Here's how the part is built. I have some questions about the finished solid (model axes, mm). Face numbers are marked on the shaded views. A direction names the side the tool comes from. Round coordinates to 2 decimals unless told otherwise and drop trailing zeros. Order: outer loops, then holes, each group sorted by start corner. A loop starts at its lowest first (then second) coordinate and runs counter-clockwise, first axis right, second up. Notation, with made-up numbers: (60, 11) - (79, 11) arc R21 ccw to (79, 16) - close; hole circle Ø9 at (49.25, 13). An arc over 180 degrees is marked (long way). Answer as a JSON object with one key per item and string values.
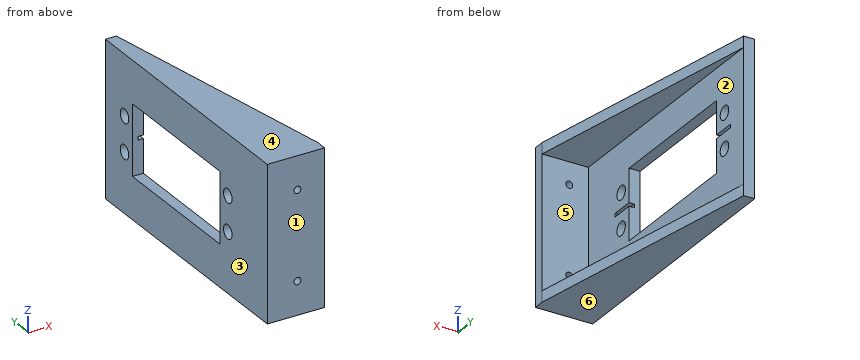
```python
from build123d import *

# Parameters (mm, degrees)
BOSS_EXTRUDE1_DEPTH = 22.225
BOSS_EXTRUDE2_DEPTH = 3.175
SKETCH4_R           = 1.000000032
CUT_EXTRUDE2_DEPTH  = 4.175
SKETCH5_R           = 2.000000064
CUT_EXTRUDE3_DEPTH  = 4.175
SKETCH6_W           = 20.253999878
SKETCH6_H           = 41.153999988
CUT_EXTRUDE4_DEPTH  = 4.175
SKETCH7_W           = 1.500000048
SKETCH7_H           = 1.000000032
CUT_EXTRUDE5_DEPTH  = 6.604
CUT_EXTRUDE6_START  = 41.154
SKETCH7_2_W         = 1.500000048
SKETCH7_2_H         = 1.000000032
CUT_EXTRUDE6_DEPTH  = 6.604


with BuildPart() as part:
    # Sketch1 → Boss-Extrude1 (new body, symmetric)
    with BuildSketch(Plane.XY):
        Polygon((0, 0), (0, 76.2), (3.175, 76.2), (3.175, 3.175), (16.51, 3.175), (16.51, 0), align=None)
    extrude(amount=BOSS_EXTRUDE1_DEPTH, both=True)

    # Sketch3 → Boss-Extrude2 (add)
    with BuildSketch(Plane.XY.offset(22.225)):
        Polygon((3.175, 76.2), (16.51, 3.175), (3.175, 3.175), align=None)
    boss_extrude2 = extrude(amount=-BOSS_EXTRUDE2_DEPTH)

    # Mirror1: Boss-Extrude2 across plane
    add(boss_extrude2.mirror(Plane.XY))

    # Sketch4 → Cut-Extrude2 (cut, through all)
    with BuildSketch(Plane(origin=(0, 3.175, 0), x_dir=(1, 0, 0), z_dir=(0, 1, 0))):
        with Locations((8.679999912, 12.7)):
            Circle(SKETCH4_R)
        with Locations((8.679999912, -12.7)):
            Circle(SKETCH4_R)
    extrude(amount=-CUT_EXTRUDE2_DEPTH, mode=Mode.SUBTRACT)

    # Sketch5 → Cut-Extrude3 (cut, through all)
    with BuildSketch(Plane(origin=(3.175, 0, 0), x_dir=(0, 0, -1), z_dir=(1, 0, 0))):
        with Locations((-4.953, 18.574999934)):
            Circle(SKETCH5_R)
        with Locations((5.047000066, 18.574999934)):
            Circle(SKETCH5_R)
        with Locations((-4.953, 67.175000016)):
            Circle(SKETCH5_R)
        with Locations((5.047000066, 67.175000016)):
            Circle(SKETCH5_R)
    extrude(amount=-CUT_EXTRUDE3_DEPTH, mode=Mode.SUBTRACT)

    # Sketch6 → Cut-Extrude4 (cut, through all)
    with BuildSketch(Plane(origin=(3.175, 0, 0), x_dir=(0, 0, -1), z_dir=(1, 0, 0))):
        with Locations((0.047000033, 42.874999975)):
            Rectangle(SKETCH6_W, SKETCH6_H)
    extrude(amount=-CUT_EXTRUDE4_DEPTH, mode=Mode.SUBTRACT)

    # Sketch7 → Cut-Extrude5 (cut)
    with BuildSketch(Plane.XZ.offset(-63.451999969)):
        with Locations((2.424999976, 0)):
            Rectangle(SKETCH7_W, SKETCH7_H)
    extrude(amount=-CUT_EXTRUDE5_DEPTH, mode=Mode.SUBTRACT)

    # Sketch7<2> → Cut-Extrude6 (cut)
    with BuildSketch(Plane.XZ.offset(-63.451999969).offset(CUT_EXTRUDE6_START)):
        with Locations((2.424999976, 0)):
            Rectangle(SKETCH7_2_W, SKETCH7_2_H)
    extrude(amount=CUT_EXTRUDE6_DEPTH, mode=Mode.SUBTRACT)


solid = part.part
```
1. Imagine slicing it at C-C (z = 12.7). List the corners of the cut face in (x, y) for me (3 decimals).
Responses:
{"outline": "(0, 0) - (7.68, 0) - (7.68, 3.175) - (3.175, 3.175) - (3.175, 76.2) - (0, 76.2) - close; (9.68, 0) - (16.51, 0) - (16.51, 3.175) - (9.68, 3.175) - close"}
2. For P1, Ø1.1, axis at y = 66, z = 0, coming from the +X side (3 decimals); P2, Ø3, axis at x = 8.68, z = 12.7, coming from the +Y side (3 decimals); P3, Ø0.8, axis at y = 20, z = 0, coming from the +X side (3 decimals), each with a flat end and sliding along its axis, tell me the tip position at first contact or that it passes through.
Responses:
{"P1": "x = 3.175", "P2": "y = 3.175", "P3": "x = 1.675"}
3. Thinking about a two-plate mould opening in Z: for the marked faces 3, 4, 5 and 6, which applies, pulls with the +Z half, pulls with the -Z half, needs draft (parallel to the pull), parting line crosses it, or undercut?
Responses:
{"face 3": "needs draft", "face 4": "pulls with the +Z half", "face 5": "undercut", "face 6": "pulls with the -Z half"}
4. Imagine slicing it at D-D (x = 8.68). List the corners of the cut face in (y, z) for me (3 decimals), plus the area to 3 significant figures.
Responses:
{"outline": "(0, -22.225) - (46.054, -22.225) - (46.054, -19.05) - (3.175, -19.05) - (3.175, -13.7) - (0, -13.7) - close; (0, -11.7) - (3.175, -11.7) - (3.175, 11.7) - (0, 11.7) - close; (0, 13.7) - (3.175, 13.7) - (3.175, 19.05) - (46.054, 19.05) - (46.054, 22.225) - (0, 22.225) - close", "area": "401 mm2"}
5. Imagine slicing it at A-A (z = -5). List the corners of the cut face in (x, y) for me (3 decimals).
Responses:
{"outline": "(0, 0) - (16.51, 0) - (16.51, 3.175) - (3.175, 3.175) - (3.175, 16.576) - (0, 16.576) - close; (0, 20.574) - (3.175, 20.574) - (3.175, 22.298) - (0, 22.298) - close; (0, 63.452) - (3.175, 63.452) - (3.175, 65.176) - (0, 65.176) - close; (0, 69.174) - (3.175, 69.174) - (3.175, 76.2) - (0, 76.2) - close"}
6. For the marked faces 1 and 2, which set-ups out of +Z, -Z, +X, -X, +Y, -Y let a thin tool reach every point of the face, with its end or its side?
Responses:
{"face 1": "+Z, -Z, +X, -X, -Y", "face 2": "+X, +Y"}
7. If I drill on L1, parallel to Z at x = 8.68, y = 2 (3 decimals); L2, parallel to X at y = 1.1, z = 12.7; L3, parallel to Y at x = 2, z = -9.5, over which ranges is the centre line in solid material (lowest first)? Write a range as [from, to].
Responses:
{"L1": "[-22.225, -13.7], [-11.7, 11.7], [13.7, 22.225]", "L2": "[0, 7.68], [9.68, 16.51]", "L3": "[0, 22.3], [63.45, 76.2]"}
8. Imagine slicing it at B-B (y = 31). List the corners of the cut face in (x, z) for me (3 decimals).
Responses:
{"outline": "(0, -22.225) - (11.429, -22.225) - (11.429, -19.05) - (3.175, -19.05) - (3.175, -10.174) - (0, -10.174) - close; (0, 10.08) - (3.175, 10.08) - (3.175, 19.05) - (11.429, 19.05) - (11.429, 22.225) - (0, 22.225) - close"}
